Verification items for the finished model (mm, model axes). A direction names the side the tool comes from. Coordinates: 2 decimals unless noted, no trailing zeros. Write each loop counter-clockwise with the first axis right and the second up, starting at its lowest first coordinate (ties: lowest second). Pieces come first, ordered by that corner, then holes. Notation, with made-up numbers: (59, 63.25) - (94, 63.25) arc R31 cw to (94, 98.25) - close; hole circle Ø8 at (46.25, -38.75). An arc over 180 degrees is marked (long way). Use one line per item in the form item = value. Start each with the question number.
(1) Gauge pin test, flat ends, axial feed: pin 1 Ø3 at (y, z) = (5, -7) entering from -X; pin 2 Ø4 at (x, z) = (-13, 8.5) entering from +Y; pin 3 Ø8 at (x, y) = (22, -5.5) entering from -Z. Record the tip position at first contact, or that the pin passes through.
(2) Sectioned sample at D-D (x = 14.5). Record the cut outline in (y, z).
(3) Material ranges on line 1 (Z direction, x = 20.5, y = 0.5); line 2 (X direction, y = -9, z = 4.5); line 3 (Y direction, x = -16.5, z = 0.75), recorded low to high. Write a range as [from, to].
(4) Sectioned sample at A-A (y = 0). Record the cut outline in (x, z).
(5) Sectioned sample at C-C (x = -34). Record the cut outline in (y, z).
(6) Tool access check on faces 1 (the flat face through (-40, 0, 0)), 2 (the cylindrical face through (-29.62, 7.81, -1.73)), 3 (the flat face through (21, 8, -2)). Record the directions out of +Z, -Z, +X, -X, +Y, -Y that give a thin tool (end or side, any length) a straight path to the whole face; none if there is none.
from build123d import *

# Parameters (mm, degrees)
CHAMFER_1_SIZE = 2


with BuildPart() as part:
    # 草圖1 → 旋轉1 (revolve)
    with BuildSketch(Plane.XY, mode=Mode.PRIVATE) as revolve_1_sk:
        Polygon((0, 0), (0, 11), (21, 11), (21, 8), (40, 8), (40, 0), align=None)
    revolve(revolve_1_sk.sketch.rotate(Axis((0, 0, 0), (1, 0, 0)), 90), axis=Axis((0, 0, 0), (1, 0, 0)))

    # 導角1
    chamfer_1_edges = [part.edges().sort_by_distance(p)[0] for p in [
        (40, 0, -8),
    ]]
    chamfer(chamfer_1_edges, length=CHAMFER_1_SIZE)

    # 鏡射1: part across plane


with BuildPart() as part_1:
    add(part.part)
    add(part.part.mirror(Plane(origin=(0, 0, 0), x_dir=(0, 0, 1), z_dir=(1, 0, 0))))


solid = part_1.part
Answers below:
q1.pin_1 = -38.9
q1.pin_2 = 8.87
q1.pin_3 = -10.88
q2.outline = circle Ø22 at (0, 0)
q3.line_1 = [-10.99, 10.99]
q3.line_2 = [-21, 21]
q3.line_3 = [-10.97, 10.97]
q4.outline = (-40, -6) - (-38, -8) - (-21, -8) - (-21, -11) - (21, -11) - (21, -8) - (38, -8) - (40, -6) - (40, 6) - (38, 8) - (21, 8) - (21, 11) - (-21, 11) - (-21, 8) - (-38, 8) - (-40, 6) - close
q5.outline = circle Ø16 at (0, 0)
q6.face_1 = +Z, -Z, -X, +Y, -Y
q6.face_2 = -X
q6.face_3 = +X
